```python
from build123d import *

# Parameters (mm, degrees)
SKETCH_1_W      = 20.32
SKETCH_1_H      = 11.43
SKETCH_1_R      = 1.905
SKETCH_1_R_2    = 0.381
EXTRUDE_1_DEPTH = 1.5


with BuildPart() as part:
    # 스케치1 → 보스-돌출1 (new body)
    with BuildSketch(Plane(origin=(0, 0, 0), x_dir=(1, 0, 0), z_dir=(0, 1, 0))):
        Rectangle(SKETCH_1_W, SKETCH_1_H)
        with Locations((-7.62, -3.175)):
            Circle(SKETCH_1_R, mode=Mode.SUBTRACT)
        with Locations((7.62, -3.175)):
            Circle(SKETCH_1_R, mode=Mode.SUBTRACT)
        with Locations((5.08, 4.445)):
            Circle(SKETCH_1_R_2, mode=Mode.SUBTRACT)
        with Locations((2.54, 4.445)):
            Circle(SKETCH_1_R_2, mode=Mode.SUBTRACT)
        with Locations((-2.54, 4.445)):
            Circle(SKETCH_1_R_2, mode=Mode.SUBTRACT)
        with Locations((-5.08, 4.445)):
            Circle(SKETCH_1_R_2, mode=Mode.SUBTRACT)
        with Locations((0, 4.445)):
            Circle(SKETCH_1_R_2, mode=Mode.SUBTRACT)
    extrude(amount=EXTRUDE_1_DEPTH)


solid = part.part
```
Model file for the job. Use its own axes, mm. Coordinates: 2 decimals unless noted, no trailing zeros. Write each loop counter-clockwise with the first axis right and the second up, starting at its lowest first coordinate (ties: lowest second). Pieces come first, ordered by that corner, then holes. Notation, with made-up numbers: (3, 67.25) - (59, 67.25) arc R9 ccw to (59, 78.25) - close; hole circle Ø6 at (-17.5, 0). An arc over 180 degrees is marked (long way). One line per item, written item: value. Start each with the question number.
1. Slice it at B-B (y = 0.75). Write the cut outline in (x, z) (3 decimals).
2. Mould opens along X. For faces 1 (the flat face through (-10.16, 1, 0)), 2 (the cylindrical face through (9.38, 0.74, 3.9)), 3 (the flat face through (0, 1.5, 0)) say: released by +X, released by -X, zero draft, split by the parting line, or undercut.
3. Probe line 1 (X direction, y = 0.1, z = -4.5); line 2 (X direction, y = 1.05, z = 4.5); line 3 (X direction, y = 0.9, z = 4). List the from-to ranges inside material, lowest first. Write a range as from..to.
4. Slice it at C-C (x = 2.54). Write the cut outline in (y, z) (3 decimals).
5. Slice it at A-A (x = 7.62). Write the cut outline in (y, z) (3 decimals).
6. Flat gauge pins, fed straight in: pin 1 (4.5 mm diameter, centred on x = -7.62, z = 3.175, fed in from -Y); pin 2 (3 mm diameter, centred on x = 7.62, z = 3.175, fed in from +Y) (3 decimals). Where does each tip first touch, or does it go through?
Answers below:
1. outline: (-10.16, -5.715) - (10.16, -5.715) - (10.16, 5.715) - (-10.16, 5.715) - close; hole circle Ø3.81 at (-7.62, 3.175); hole circle Ø0.762 at (-5.08, -4.445); hole circle Ø0.762 at (-2.54, -4.445); hole circle Ø0.762 at (0, -4.445); hole circle Ø0.762 at (2.54, -4.445); hole circle Ø0.762 at (5.08, -4.445); hole circle Ø3.81 at (7.62, 3.175)
2. face 1: released by -X
2. face 2: undercut
2. face 3: zero draft
3. line 1: x = -10.16..-5.46, -4.7..-2.92, -2.16..-0.38, 0.38..2.16, 2.92..4.7, 5.46..10.16
3. line 2: x = -10.16..-8.99, -6.25..6.25, 8.99..10.16
3. line 3: x = -10.16..-9.34, -5.9..5.9, 9.34..10.16
4. outline: (0, -5.715) - (1.5, -5.715) - (1.5, -4.826) - (0, -4.826) - close; (0, -4.064) - (1.5, -4.064) - (1.5, 5.715) - (0, 5.715) - close
5. outline: (0, -5.715) - (1.5, -5.715) - (1.5, 1.27) - (0, 1.27) - close; (0, 5.08) - (1.5, 5.08) - (1.5, 5.715) - (0, 5.715) - close
6. pin 1: stops at y = 0
6. pin 2: passes through
